from build123d import *

# Parameters (mm, degrees)
F0_W     = 76.2
F0_H     = 38.1
F1_DEPTH = 876.3
F2_R     = 6.35
F3_DEPTH = 876.3
F4_R     = 6.35
F5_DEPTH = 876.3


with BuildPart() as f1:
    # F0 (on Front) → F1 (new body)
    with BuildSketch(Plane.XZ):
        with Locations((-70.408251, 44.989463)):
            Rectangle(F0_W, F0_H)
    extrude(amount=F1_DEPTH)

    # F2 (on face) → F3 (cut)
    with BuildSketch(Plane.XZ.offset(876.3)):
        with Locations((-70.408251, 64.039463)):
            Circle(F2_R)
    extrude(amount=-F3_DEPTH, mode=Mode.SUBTRACT)

    # F4 (on face) → F5 (cut)
    with BuildSketch(Plane.XZ.offset(876.3)):
        with Locations((-32.308251, 44.989463)):
            Circle(F4_R)
        with Locations((-108.508251, 44.989463)):
            Circle(F4_R)
        with Locations((-70.408251, 25.939463)):
            Circle(F4_R)
    extrude(amount=-F5_DEPTH, mode=Mode.SUBTRACT)


solid = f1.part
Input: part model. Units: mm. Frame: model coordinates. Give positions to 0.01 mm unless a question says otherwise; leave off trailing zeros. Write each loop counter-clockwise with the first axis right and the second up, starting at its lowest first coordinate (ties: lowest second). Pieces come first, ordered by that corner, then holes.
Q1. Section A-A, the plane y = -223. Output: boundary loops of the cut face in (x, z).
Q2. First-contact query: P1, Ø8, axis at y = -517.5, z = 49.5, coming from the -X side; P2, Ø1.5, axis at y = -505.5, z = 47.5, coming from the +X side; P3, Ø6, axis at y = -365.5, z = 46.5, coming from the -X side. Flat tips, straight axial feed; report the tip coordinate or a pass-through.
Q3. Material intervals for probe 1 along X at (y, z) = (-109.5, 28.5); probe 2 along Z at (x, y) = (-37.5, -406); probe 3 along Z at (x, y) = (-103, -721.5), sorted ascending.
Filled in:
1. outline: (-108.51, 25.94) - (-76.76, 25.94) arc R6.35 cw to (-64.06, 25.94) - (-32.31, 25.94) - (-32.31, 38.64) arc R6.35 cw to (-32.31, 51.34) - (-32.31, 64.04) - (-64.06, 64.04) arc R6.35 cw to (-76.76, 64.04) - (-108.51, 64.04) - (-108.51, 51.34) arc R6.35 cw to (-108.51, 38.64) - close
2. P1: stops at x = -108.51
2. P2: stops at x = -37.76
2. P3: stops at x = -104.04
3. probe 1: x = -108.51 to -76.22, -64.6 to -32.31
3. probe 2: z = 25.94 to 41.33, 48.65 to 64.04
3. probe 3: z = 25.94 to 41.83, 48.15 to 64.04
